from build123d import *

# Parameters (mm, degrees)
EXTRUDE_1_DEPTH      = 2
EXTRUDE_1_DEPTH_BACK = 5
SKETCH_1_R           = 8
SKETCH_2_R           = 6
EXTRUDE_2_DEPTH      = 16
SKETCH_3_R           = 7.5
EXTRUDE_3_DEPTH      = 2
SKETCH_4_R           = 3
CUT_EXTRUDE_1_DEPTH  = 34


with BuildPart() as part:
    # 草图1 → 凸台-拉伸1 (new, two sides: drawn at the far end of the back side and taken through both)
    with BuildSketch(Plane(origin=(0, 0, 0), x_dir=(1, 0, 0), z_dir=(0, 1, 0)).offset(-EXTRUDE_1_DEPTH_BACK)):
        with Locations(Location((0, 0, 0), (0, 0, 270))):
            Circle(SKETCH_1_R)
    extrude(amount=EXTRUDE_1_DEPTH + EXTRUDE_1_DEPTH_BACK)

    # 草图2 → 凸台-拉伸2 (add)
    with BuildSketch(Plane(origin=(0, 2, 0), x_dir=(1, 0, 0), z_dir=(0, 1, 0))):
        with Locations(Location((0, 0, 0), (0, 0, 270))):
            Circle(SKETCH_2_R)
    extrude(amount=EXTRUDE_2_DEPTH)

    # 草图3 → 凸台-拉伸3 (add)
    with BuildSketch(Plane(origin=(0, 18, 0), x_dir=(1, 0, 0), z_dir=(0, 1, 0))):
        with Locations(Location((0, 0, 0), (0, 0, 270))):
            Circle(SKETCH_3_R)
    extrude(amount=EXTRUDE_3_DEPTH)

    # 草图4 → 切除-拉伸1 (cut)
    with BuildSketch(Plane(origin=(0, 20, 0), x_dir=(1, 0, 0), z_dir=(0, 1, 0))):
        with Locations(Location((0, 0, 0), (0, 0, 270))):
            Circle(SKETCH_4_R)
    extrude(amount=-CUT_EXTRUDE_1_DEPTH, mode=Mode.SUBTRACT)


solid = part.part
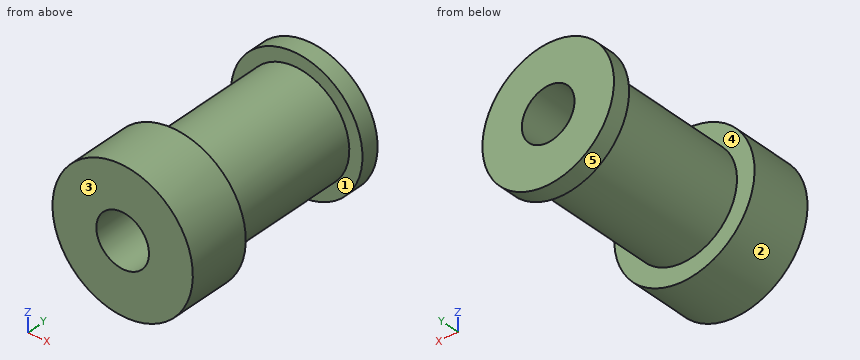
Part model, mm, in its own coordinate system. Face numbers are marked on the shaded views. A direction names the side the tool comes from. Give positions to 0.01 mm unless a question says otherwise; leave off trailing zeros. Loops run counter-clockwise (first coordinate to the right, second up) from the corner with the lowest first, then second, coordinate; pieces in that order, holes last.
(1) Pull direction Y, two halves, no side cores. Call the marked faces 3, 4 and 5: pulls with the +Y half, pulls with the -Y half, needs draft (parallel to the pull), parting line crosses it, or undercut.
Return value:
face 3: pulls with the -Y half
face 4: undercut
face 5: needs draft
(2) 3-axis set-ups, long thin cutter, end or side, ignore diameter. For the marked faces 1 and 2: which of +Z, -Z, +X, -X, +Y, -Y reach the whole face in a straight line?
Return value:
face 1: none
face 2: +Y, -Y
(3) Band-saw the part on A-A (x = 0). Write the cut outline in (y, z), and give its area (3 significant figures).
Return value:
outline: (-5, -8) - (2, -8) - (2, -6) - (18, -6) - (18, -7.5) - (20, -7.5) - (20, -3) - (-5, -3) - close; (-5, 3) - (20, 3) - (20, 7.5) - (18, 7.5) - (18, 6) - (2, 6) - (2, 8) - (-5, 8) - close
area: 184 mm2
(4) Band-saw the part on C-C (y = 5). Write the cut outline in (x, z), and give its area (3 significant figures).
Return value:
outline: circle Ø12 at (0, 0); hole circle Ø6 at (0, 0)
area: 84.8 mm2
(5) Band-saw the part on B-B (z = 0). Write the cut outline in (x, y).
Return value:
outline: (-8, -5) - (-3, -5) - (-3, 20) - (-7.5, 20) - (-7.5, 18) - (-6, 18) - (-6, 2) - (-8, 2) - close; (3, -5) - (8, -5) - (8, 2) - (6, 2) - (6, 18) - (7.5, 18) - (7.5, 20) - (3, 20) - close
(6) Band-saw the part on D-D (x = 3.75). Write the cut outline in (y, z).
Return value:
outline: (-5, -7.07) - (2, -7.07) - (2, -4.68) - (18, -4.68) - (18, -6.5) - (20, -6.5) - (20, 6.5) - (18, 6.5) - (18, 4.68) - (2, 4.68) - (2, 7.07) - (-5, 7.07) - close
(7) Pin check, flat tips, straight feed: pin 1 (5 mm diameter, centred on y = -1.5, z = -4.5, fed in from +X); pin 2 (3 mm diameter, centred on x = -1.5, y = 13.5, fed in from +Z); pin 3 (6 mm diameter, centred on y = 12.5, z = -1.5, fed in from +X). Stop position of each tip, or through.
Return value:
pin 1: stops at x = 7.75
pin 2: stops at z = 6
pin 3: stops at x = 6
(8) Drill centre lines: line 1 along Y through (x, z) = (6.5, -1.75); line 2 along X through (y, z) = (8.5, 0); line 3 along Y through (x, z) = (-3, 7.25). Where is each one in solid material? Low to high.
Return value:
line 1: y = -5 to 2, 18 to 20
line 2: x = -6 to -3, 3 to 6
line 3: y = -5 to 2
